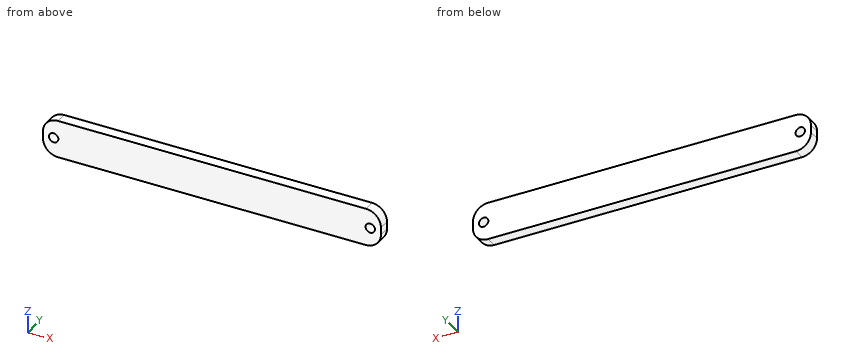
```python
from build123d import *

# Parameters (mm, degrees)
SKETCH1_W           = 114.3
SKETCH1_H           = 12.7
EXTRUDE_THIN1_DEPTH = 3.81
FILLET1_R           = 5.08
SKETCH3_R           = 1.5875
CUT_EXTRUDE1_DEPTH  = 3.81


with BuildPart() as part:
    # Sketch1 → Extrude-Thin1 (new body)
    with BuildSketch(Plane(origin=(0, 0, 0), x_dir=(1, 0, 0), z_dir=(0, 1, 0))):
        with Locations((0, -6.35)):
            Rectangle(SKETCH1_W, SKETCH1_H)
    extrude(amount=EXTRUDE_THIN1_DEPTH)

    # Fillet1
    fillet1_edges = [part.edges().sort_by_distance(p)[0] for p in [
        (-57.15, 1.905, 12.7),
        (-57.15, 1.905, 0),
        (57.15, 1.905, 0),
        (57.15, 1.905, 12.7),
    ]]
    fillet(fillet1_edges, radius=FILLET1_R)

    # Sketch3 → Cut-Extrude1 (cut)
    with BuildSketch(Plane(origin=(0, 3.81, 0), x_dir=(1, 0, 0), z_dir=(0, 1, 0))):
        with Locations((53.54685275, -6.35)):
            Circle(SKETCH3_R)
    cut_extrude1 = extrude(amount=-CUT_EXTRUDE1_DEPTH, mode=Mode.SUBTRACT)

    # Mirror1: Cut-Extrude1 across plane
    add(cut_extrude1.mirror(Plane(origin=(0, 0, 0), x_dir=(0, 0, 1), z_dir=(1, 0, 0))), mode=Mode.SUBTRACT)


solid = part.part
```
Can you work these out from the model? Positions are in its coordinate system, mm. Round coordinates to 2 decimals unless told otherwise and drop trailing zeros. Order: outer loops, then holes, each group sorted by start corner. A loop starts at its lowest first (then second) coordinate and runs counter-clockwise, first axis right, second up.
(1) I'm going to push a flat-ended pin straight in: pin 1 (1 mm diameter, centred on y = 1, z = 2, fed in from -X). Where does the tip first touch, or does it pass through?
Results are:
pin 1: stops at x = -56.45
(2) If we section it at A-A (z = 6.35): Please give me the cut outline in (x, y), plus the area to 3 significant figures.
Results are:
outline: (-57.15, 0) - (-55.13, 0) - (-55.13, 3.81) - (-57.15, 3.81) - close; (-51.96, 0) - (51.96, 0) - (51.96, 3.81) - (-51.96, 3.81) - close; (55.13, 0) - (57.15, 0) - (57.15, 3.81) - (55.13, 3.81) - close
area: 411 mm2
(3) If I drill on L1, parallel to X at y = 2.25, z = 6.35; L2, parallel to X at y = 0.85, z = 5.5; L3, parallel to X at y = 2.35, z = 1.25, over which ranges is the centre line in solid material (lowest first)?
Results are:
L1: x = -57.15 to -55.13, -51.96 to 51.96, 55.13 to 57.15
L2: x = -57.15 to -54.89, -52.21 to 52.21, 54.89 to 57.15
L3: x = -55.41 to 55.41
(4) If we section it at C-C (z = 1.5): Please give me the cut outline in (x, y).
Results are:
outline: (-55.67, 0) - (55.67, 0) - (55.67, 3.81) - (-55.67, 3.81) - close
(5) If we section it at B-B (y = 2.4): Count the separate pieces of the cut face and the enclosed holes in it, plus the area to 3 significant figures.
Results are:
separate pieces: 1
enclosed holes: 2
area: 1,410 mm2
